from build123d import *

# Parameters (mm, degrees)
CYLINDER003_R     = 0.75
CYLINDER003_DEPTH = 10
ARRAY_COUNT       = 4
CYLINDER002_R     = 4.35
CYLINDER002_DEPTH = 10
CYLINDER001_R     = 10.9
CYLINDER001_DEPTH = 10
TORUS_R           = 1.5
CYLINDER_R        = 28
CYLINDER_DEPTH    = 6


with BuildPart() as array:
    # Cylinder003 → Cylinder003 (new body)
    with BuildSketch(Plane(origin=(7.3, 0, -2), x_dir=(1, 0, 0), z_dir=(0, 0, 1))):
        Circle(CYLINDER003_R)
    extrude(amount=CYLINDER003_DEPTH)

    # Array: Array ×4 about axis
    array_axis = Axis((0, 0, 0), (0, 0, 1))


with BuildPart() as array_1:
    add(array.part)
    for i in range(1, ARRAY_COUNT):
        add(array.part.rotate(array_axis, i * 360 / ARRAY_COUNT))


with BuildPart() as hueco_eje:
    # Cylinder002 → Cylinder002 (new body)
    with BuildSketch(Plane.XY.offset(-2)):
        Circle(CYLINDER002_R)
    extrude(amount=CYLINDER002_DEPTH)


with BuildPart() as corona_servo:
    # Cylinder001 → Cylinder001 (new body)
    with BuildSketch(Plane.XY.offset(2)):
        Circle(CYLINDER001_R)
    extrude(amount=CYLINDER001_DEPTH)


with BuildPart() as obj1:
    # Torus → Torus (revolve)
    with BuildSketch(Plane(origin=(0, 0, 3), x_dir=(1, 0, 0), z_dir=(0, -1, 0))):
        with Locations((28, 0)):
            Circle(TORUS_R)
    revolve(axis=Axis((0, 0, 3), (0, 0, 1)))


with BuildPart() as obj2:
    # Cylinder → Cylinder (new body)
    with BuildSketch(Plane.XY):
        Circle(CYLINDER_R)
    extrude(amount=CYLINDER_DEPTH)

    # Cut: cut obj1
    add(obj1.part, mode=Mode.SUBTRACT)

    # Cut001: cut Corona_servo
    add(corona_servo.part, mode=Mode.SUBTRACT)

    # Cut002: cut Hueco_eje
    add(hueco_eje.part, mode=Mode.SUBTRACT)

    # Cut003: cut Array
    add(array_1.part, mode=Mode.SUBTRACT)


solid = obj2.part
Geometry check sheet. Reference: the model listing, model coordinates, mm. A direction names the side the tool comes from. Give positions to 0.01 mm unless a question says otherwise; leave off trailing zeros. Write each loop counter-clockwise with the first axis right and the second up, starting at its lowest first coordinate (ties: lowest second). Pieces come first, ordered by that corner, then holes. Notation, with made-up numbers: M 28.5,43 L 46.5,43 A24 cw 46.5,56 Z; hole C -17,86 d1. An arc over 180 degrees is marked long. Answer as CSV lines item,"result". Start each with the question number.
Q1. Tool access check on faces 1 (the face through (10.4, 3.27, 3.97)), 2 (the face through (-0.03, 6.55, 0.99)). Record the directions out of +Z, -Z, +X, -X, +Y, -Y that give a thin tool (end or side, any length) a straight path to the whole face; none if there is none.
Q2. Release check for a two-part mould opening along X. For faces 3 (the face through (-0.943, -4.247, 0.986)), 4 (the face through (25.865, -10.724, 0.74)), 5 (the face through (0, -12, 6)) record: pulls with the +X half, pulls with the -X half, needs draft (parallel to the pull), parting line crosses it, or undercut.
Q3. Section check C-C, the plane z = 3.1. Record the cut outline in (x, y).
Q4. Go/stop test with flat-tipped pins: pin 1 (2 mm diameter, centred on x = 7.3, y = 0, fed in from +Z); pin 2 (2 mm diameter, centred on x = 9.5, z = 1.5, fed in from +Y); pin 3 (1 mm diameter, centred on y = 17.5, z = 1, fed in from -X). Record where each tip stops, or that it passes through.
Q5. Material ranges on L1, parallel to Z at x = 4, y = -4.5; L2, parallel to X at y = 5, z = 2.6; L3, parallel to X at y = 9.5, z = 3.05, recorded low to high.
Q6. Section check A-A, the plane x = 0. Record the cut outline in (y, z).
Geometry says:
1,face 1,"+Z"
1,face 2,"+Z, -Z"
2,face 3,"undercut"
2,face 4,"parting line crosses it"
2,face 5,"needs draft"
3,outline,"C 0,0 d53.01; hole C 0,0 d21.8"
4,pin 1,"z = 2"
4,pin 2,"y = 26.68"
4,pin 3,"x = -22.25"
5,L1,"0 to 2"
5,L2,"-26.08 to -9.69, 9.69 to 26.08"
5,L3,"-24.74 to -5.34, 5.34 to 24.74"
6,outline,"M -28,0 L -8.05,0 L -8.05,2 L -10.9,2 L -10.9,6 L -28,6 L -28,4.5 A1.5 cw -28,1.5 Z; M -6.55,0 L -4.35,0 L -4.35,2 L -6.55,2 Z; M 4.35,0 L 6.55,0 L 6.55,2 L 4.35,2 Z; M 8.05,0 L 28,0 L 28,1.5 A1.5 cw 28,4.5 L 28,6 L 10.9,6 L 10.9,2 L 8.05,2 Z"
